```python
from build123d import *

# Parameters (mm, degrees)
SKETCH1_R           = 26
BOSS_EXTRUDE1_DEPTH = 2
SKETCH2_R           = 14.75
CUT_EXTRUDE1_DEPTH  = 37.823905279
SKETCH3_R           = 1.7
CUT_EXTRUDE2_DEPTH  = 37.823905279


with BuildPart() as part:
    # Sketch1 → Boss-Extrude1 (new body)
    with BuildSketch(Plane.YZ):
        with Locations(Location((0, 0, 0), (0, 0, 270))):
            Circle(SKETCH1_R)
    extrude(amount=BOSS_EXTRUDE1_DEPTH)

    # Sketch2 → Cut-Extrude1 (cut, through all)
    with BuildSketch(Plane.YZ.offset(2)):
        with Locations(Location((0, 0, 0), (0, 0, 270))):
            Circle(SKETCH2_R)
    extrude(amount=-CUT_EXTRUDE1_DEPTH, mode=Mode.SUBTRACT)

    # Sketch3 → Cut-Extrude2 (cut, through all)
    with BuildSketch(Plane.YZ.offset(2)):
        with Locations(Location((22.5, 0, 0), (0, 0, 270))):
            Circle(SKETCH3_R)
        with Locations(Location((-11.25, -19.485571585, 0), (0, 0, 270))):
            Circle(SKETCH3_R)
        with Locations(Location((-11.25, 19.485571585, 0), (0, 0, 270))):
            Circle(SKETCH3_R)
    extrude(amount=-CUT_EXTRUDE2_DEPTH, mode=Mode.SUBTRACT)


solid = part.part
```
Verification items for the finished model (mm, model axes). Coordinates: 2 decimals unless noted, no trailing zeros. Write each loop counter-clockwise with the first axis right and the second up, starting at its lowest first coordinate (ties: lowest second). Pieces come first, ordered by that corner, then holes. Notation, with made-up numbers: M 81,22.25 L 117,22.25 A24 cw 117,58.25 Z; hole C -5,2.25 d10. An arc over 180 degrees is marked long. Answer as a JSON object with one key per item and string values. Group by question number.
(1) Cross-section at D-D, the plane z = -11.5. Record the cut outline in (x, y), and give its area (3 significant figures).
(2) Cross-section at C-C, the plane y = 22.5. Record the cut outline in (x, z).
(3) Cross-section at B-B, the plane x = 1.5. Record the cut outline in (y, z), and give its area (3 significant figures).
(4) Release check for a two-part mould opening along Y. For faces 1 (the face through (1.014, -12.284, -18.137)), 2 (the face through (0.986, -15.821, 20.633)), 3 (the face through (0, -11, -11)) record: +Y half, -Y half, draft (parallel to the pull), parting line (faces both ways), or undercut.
(5) Cross-section at A-A, the plane z = 0. Record the cut outline in (x, y).
(6) Material ranges on line 1 (Y direction, x = 0.8, z = 0); line 2 (Y direction, x = 0.85, z = 1); line 3 (Z direction, x = 1.8, y = -4), recorded low to high.
(7) Gauge pin test, flat end, axial feed: pin 1 (3 mm diameter, centred on y = -11.25, z = -19.49, fed in from -X). Record the tip position at first contact, or that the pin passes through.
Reply:
{
 "1": {"outline": "M 0,-23.32 L 2,-23.32 L 2,-9.24 L 0,-9.24 Z; M 0,9.24 L 2,9.24 L 2,23.32 L 0,23.32 Z", "area": "56.3 mm²"},
 "2": {"outline": "M 0,-13.03 L 2,-13.03 L 2,-1.7 L 0,-1.7 Z; M 0,1.7 L 2,1.7 L 2,13.03 L 0,13.03 Z"},
 "3": {"outline": "C 0,0 d52; hole C 0,0 d29.5; hole C -11.25,-19.49 d3.4; hole C -11.25,19.49 d3.4; hole C 22.5,0 d3.4", "area": "1,410 mm²"},
 "4": {"face 1": "undercut", "face 2": "parting line", "face 3": "draft"},
 "5": {"outline": "M 0,-26 L 2,-26 L 2,-14.75 L 0,-14.75 Z; M 0,14.75 L 2,14.75 L 2,20.8 L 0,20.8 Z; M 0,24.2 L 2,24.2 L 2,26 L 0,26 Z"},
 "6": {"line 1": "-26 to -14.75, 14.75 to 20.8, 24.2 to 26", "line 2": "-25.98 to -14.72, 14.72 to 21.13, 23.87 to 25.98", "line 3": "-25.69 to -14.2, 14.2 to 25.69"},
 "7": {"pin 1": "through"}
}
